Read the model definition and answer for the solid it produces. Units are mm, in the model's axes. Coordinates: 2 decimals unless noted, no trailing zeros. Order: outer loops, then holes, each group sorted by start corner. A loop starts at its lowest first (then second) coordinate and runs counter-clockwise, first axis right, second up.
Autodesk Inventor part; units mm, degrees
ref_plane "YZ Plane" through (0, 0, 0) normal (1, 0, 0) x (0, 1, 0)
ref_plane "XZ Plane" through (0, 0, 0) normal (0, 1, 0) x (-1, 0, 0)
ref_plane "XY Plane" through (0, 0, 0) normal (0, 0, 1) x (1, 0, 0)
sketch "Sketch1" plane through (0, 0, 0) normal (0, 0, 1) x (1, 0, 0)
  line L0 (3.6554, 6.3562) -> (7.3323, 0.0125)
  line L1 (7.3323, 0.0125) -> (3.677, -6.3438)
  line L2 (3.677, -6.3438) -> (-3.6554, -6.3562)
  line L3 (-3.6554, -6.3562) -> (-7.3323, -0.0125)
  line L4 (-7.3323, -0.0125) -> (-3.677, 6.3438)
  line L5 (-3.677, 6.3438) -> (3.6554, 6.3562)
  point P0 (0, 0)
  point P1 (0, 0)
  dimension "d0" = 12.7
extrude "Extrusion1" add sketch "Sketch1" along normal blind 330.2
properties part number "CAR_035_KickerShaft" material "Aluminum 6061"
1) Flat-ended cylindrical pins translate along their axes: pin 1 Ø1 at (y, z) = (2.5, 288.5) entering from -X (3 decimals); pin 2 Ø1 at (x, z) = (-3.5, 145) entering from +Y; pin 3 Ø3 at (y, z) = (-4, 246.5) entering from +X. Find the tip coordinate at first contact, or state that the pin passes through.
A:
pin 1: stops at x = -6.175
pin 2: stops at y = 6.34
pin 3: stops at x = 5.89
2) A cutting plane is placed at A-A, the plane z = 57.5. Determine the outline of the cut face in (x, y), and give its area (3 significant figures).
A:
outline: (-7.33, -0.01) - (-3.66, -6.36) - (3.68, -6.34) - (7.33, 0.01) - (3.66, 6.36) - (-3.68, 6.34) - close
area: 140 mm2
3) A cutting plane is placed at B-B, the plane y = 3.5. Determine the outline of the cut face in (x, z), and give its area (3 significant figures).
A:
outline: (-5.31, 0) - (5.31, 0) - (5.31, 330.2) - (-5.31, 330.2) - close
area: 3,510 mm2
4) Straight lines are drawn through the part: line 1 (X direction, y = 1.75, z = 285.5); line 2 (Y direction, x = -1.75, z = 174.5). For each, find the intervals that lie inside material, in ascending order.
A:
line 1: x = -6.32 to 6.33
line 2: y = -6.35 to 6.35
